Autodesk Inventor part; units mm, degrees
ref_plane "YZ Plane" through (0, 0, 0) normal (1, 0, 0) x (0, 1, 0)
ref_plane "XZ Plane" through (0, 0, 0) normal (0, 1, 0) x (-1, 0, 0)
ref_plane "XY Plane" through (0, 0, 0) normal (0, 0, 1) x (1, 0, 0)
sketch "Sketch1" plane through (0, 0, 0) normal (0, 0, 1) x (1, 0, 0)
  line L0 (-9.525, -52.5) -> (9.525, -52.5)
  line L1 (9.525, -52.5) -> (9.525, 52.5)
  line L2 (9.525, 52.5) -> (-9.525, 52.5)
  line L3 (-9.525, 52.5) -> (-9.525, -52.5)
  line L4 (-9.525, -52.5) -> (9.525, 52.5) construction
  line L5 (9.525, -52.5) -> (-9.525, 52.5) construction
  point P0 (0, 0)
  dimension "d0" = 19.05
  dimension "d1" = 105
extrude "Extrusion1" add sketch "Sketch1" along normal blind 6.35
sketch "Sketch3" plane through (-9.525, 52.5, 0) normal (0, 1, 0) x (1, 0, 0)
  line L0 (19.05, 0) -> (0, 0)
  line L1 (0, 0) -> (0, -6.35)
  line L2 (19.05, -6.35) -> (0, -6.35)
  line L3 (19.05, 0) -> (19.05, -6.35)
  line L4 (0, 0) -> (0, -6.35)
  line L5 (0, 0) -> (19.05, -6.35)
  point P0 (9.525, 0)
  point P1 (9.525, -3.175)
hole "Hole1" at (0, 52.5, 3.175) direction (0, -1, 0) diameter 2.156 depth 8.865 tip angle 118
mirror "Mirror1" about plane through (0, 0, 0) normal (0, 1, 0) of "Hole1"
equation "\"d0\" = sensorHolderDepth"
equation "\"d2\" = acrylicThickness"
equation "\"acrylicThickness\" = 6.35"
equation "\"height\" = 127"
equation "\"width\" = 127"
equation "\"depth\" = 127"
equation "\"mirrorAngle\" = 5deg"
equation "\"detectorWidth\" = 52"
equation "\"detectorHeight\" = 52"
equation "\"mirrorThickness\" = 3.175"
equation "\"fresnelThickness\" = 0.1"
equation "\"focalLength\" = 76.2"
equation "\"ior\" = 1.49"
equation "\"centerThickness\" = 1.524"
equation "\"fresnelAngle\" = 90deg"
equation "\"fresnelEffectiveDiameter\" = 152.4"
equation "\"mirrorSuppourtWidth\" = 38.1"
equation "\"backGrooveBit\" = 4.8006"
equation "\"detectorOpeningWidth\" = 76.2"
equation "\"detectorOpeningHeight\" = 76.2"
equation "\"sensorHolderSensorHeight\" = 53.975"
equation "\"sensorHolderSensorWidth\" = 53.975"
equation "\"oRingWidth\" = 1.5875"
equation "\"sensorHolderORingID\" = 203.2"
equation "\"sensorHolderFlushORingID\" = 304.8"
equation "\"frontBackORingID\" = 419.1"
equation "\"mirrorGroove\" = 19.05"
equation "\"backMirrorGroove\" = 6.35"
equation "\"fresnelMirrorChamfer\" = 6.35"
equation "\"mirrorGrooveMill\" = 3.175"
equation "\"sensorHolderDepth\" = 19.05"
equation "\"frameAcrylicThickness\" = 9.525"
equation "\"internalAcrylicThicnkess\" = 6.35"
equation "\"internalAcrylicThickness\" = 6.35"
equation "\"aerogelClearence\" = 3.175"
equation "\"backplanePCBWidth\" = 76.2"
equation "\"backplanePostionOffsett\" = 12.7"
equation "\"backplaneHoleOffsett\" = 6.35"
equation "\"backplanePCBHeight\" = 76.2"
equation "\"moduleSlotClearence\" = 0.79375"
equation "\"plasticThickness\" = 6.35"
equation "\"aerogelHolderDepth\" = 37.30625"
properties part number "detectorSuppourt" material "ABS Plastic"
CAD build for the part. Positions are in the model's coordinates, mm. A direction names the side the tool comes from. Give positions to 0.01 mm unless a question says otherwise; leave off trailing zeros. One line per question, with ' | ' between items. Start each with the question number.
1. Probe L1, parallel to Z at x = 0, y = -46.75. List the from-to ranges inside material, lowest first. Write a range as from..to.
2. Flat gauge pins, fed straight in: pin 1 (1.9 mm diameter, centred on x = 0, z = 3.175, fed in from -Y); pin 2 (4 mm diameter, centred on x = 6, y = -28.5, fed in from -Z). Where does each tip first touch, or does it go through?
3. 3-axis set-ups, long thin cutter, end or side, ignore diameter. For faces 1 (the face through (-9.525, 1, 3)), 2 (the face through (-0.05, 48.01, 2.1)), 3 (the face through (0.05, -48.01, 2.1)): which of +Z, -Z, +X, -X, +Y, -Y reach the whole face in a straight line?
Result sheet:
1) L1: z = 0..2.1, 4.25..6.35
2) pin 1: stops at y = -43.56 | pin 2: stops at z = 0
3) face 1: +Z, -Z, -X, +Y, -Y | face 2: +Y | face 3: -Y
